Here's how the part is built. I have some questions about the finished solid (model axes, mm). Face numbers are marked on the shaded views. A direction names the side the tool comes from. Round coordinates to 2 decimals unless told otherwise and drop trailing zeros. Loops run counter-clockwise (first coordinate to the right, second up) from the corner with the lowest first, then second, coordinate; pieces in that order, holes last. Notation, with made-up numbers: M 40,22 L 92,22 A29 cw 92,51 Z; hole C -8.75,-9.75 d4. An arc over 180 degrees is marked long. Use a Markdown table: item, result.
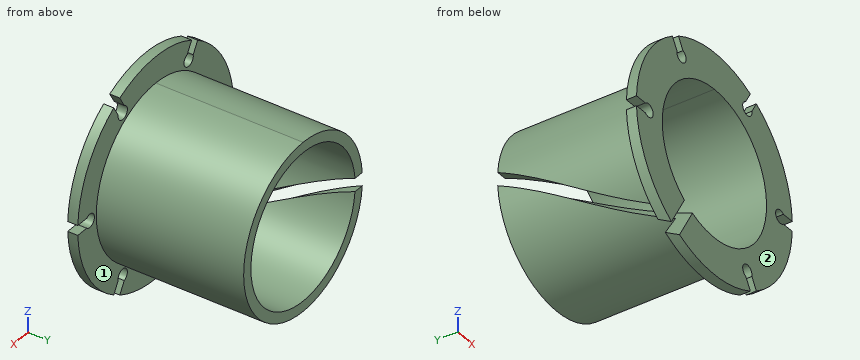
from build123d import *

# Parameters (mm, degrees)
SKETCH2_R           = 6.35
SKETCH2_R_2         = 5.5753
BOSS_EXTRUDE1_DEPTH = 11.8872
SKETCH3_R           = 8.334375
SKETCH3_R_2         = 6.35
BOSS_EXTRUDE2_DEPTH = 0.762
CUT_EXTRUDE1_DEPTH  = 17.207827995
CIRPATTERN1_COUNT   = 6


with BuildPart() as part:
    # Sketch2 → Boss-Extrude1 (new body)
    with BuildSketch(Plane(origin=(0, 0, 0), x_dir=(1, 0, 0), z_dir=(0, 1, 0))):
        with Locations(Location((0, 0, 0), (0, 0, 270))):
            Circle(SKETCH2_R)
        with Locations(Location((0, 0, 0), (0, 0, 270))):
            Circle(SKETCH2_R_2, mode=Mode.SUBTRACT)
    extrude(amount=BOSS_EXTRUDE1_DEPTH)

    # Sketch3 → Boss-Extrude2 (add)
    with BuildSketch(Plane(origin=(0, 0, 0), x_dir=(1, 0, 0), z_dir=(0, 1, 0))):
        with Locations(Location((0, 0, 0), (0, 0, 90))):
            Circle(SKETCH3_R)
        with Locations(Location((0, 0, 0), (0, 0, 270))):
            Circle(SKETCH3_R_2, mode=Mode.SUBTRACT)
    extrude(amount=BOSS_EXTRUDE2_DEPTH)

    # Sketch7 → Cut-Extrude1 (cut, through all)
    with BuildSketch(Plane(origin=(0, 0.762, 0), x_dir=(1, 0, 0), z_dir=(0, 1, 0))):
        with BuildLine():
            Line((-7.372666422, 0.372070313), (-8.334375, 0.372070312))
            Line((-8.334375, 0.372070312), (-8.334375, -0.372070312))
            Line((-8.334375, -0.372070312), (-7.372666422, -0.372070313))
            ThreePointArc((-7.372666422, -0.372070313), (-6.5484375, 0), (-7.372666422, 0.372070313))
        make_face()
    cut_extrude1 = extrude(amount=-CUT_EXTRUDE1_DEPTH, mode=Mode.SUBTRACT)

    # CirPattern1: Cut-Extrude1 ×6 about axis, 1 skipped
    cirpattern1_axis = Axis((0, 11.8872, 0), (0, -1, 0))
    add([cut_extrude1.rotate(cirpattern1_axis, i * 360 / CIRPATTERN1_COUNT) for i in range(1, CIRPATTERN1_COUNT) if i not in (1,)], mode=Mode.SUBTRACT)

    # Sketch13 → Cut-Loft1 section 0
    with BuildSketch(Plane.XZ):
        with BuildLine():
            Line((-3.206222175, -4.561152207), (-5.86681729, -9.169438125))
            Line((-5.86681729, -9.169438125), (-5.00755771, -9.665531875))
            Line((-5.00755771, -9.665531875), (-2.346962594, -5.057245957))
            Line((-2.346962594, -5.057245957), (-3.206222175, -4.561152207))
        make_face()
    # Sketch12 → Cut-Loft1 section 1
    with BuildSketch(Plane(origin=(0, 11.8872, 0), x_dir=(1, 0, 0), z_dir=(0, 1, 0))):
        with BuildLine():
            Line((-10.874375, 0.49609375), (-5.553184769, 0.49609375))
            Line((-5.553184769, 0.49609375), (-5.553184769, -0.49609375))
            Line((-5.553184769, -0.49609375), (-10.874375, -0.49609375))
            Line((-10.874375, -0.49609375), (-10.874375, 0.49609375))
        make_face()
    loft(mode=Mode.SUBTRACT)


solid = part.part
1. I need wall thicknesses on probe 1 along Z at (x, y) = (-0.25, 11.25); probe 2 along X at (y, z) = (0.25, 0); probe 3 along Y at (x, z) = (-1.5, -7.5). Which ranges of each line are inside material? Lowest first, please. Write a range as from..to.
Answer sheet:
| item | result |
|---|---|
| probe 1 | -6.35..-5.57, 5.57..6.35 |
| probe 2 | -6.55..-5.58, 5.58..6.55 |
| probe 3 | 0..0.76 |
2. Which directions (+Z, -Z, +X, -X, +Y, -Y) give clear straight access to the entire face, cutting with the end or side of a thin tool? Please do the marked faces 1 and 2.
Answer sheet:
| item | result |
|---|---|
| face 1 | +Y |
| face 2 | +Z, -Z, +X, -X, -Y |
3. Imagine slicing it at A-A, the plane x = 0.75. Write out the boundary of the cut face in (y, z).
Answer sheet:
| item | result |
|---|---|
| outline | M 0,-8.3 L 0.76,-8.3 L 0.76,-6.31 L 11.89,-6.31 L 11.89,-5.52 L 0,-5.52 Z; M 0,5.52 L 11.89,5.52 L 11.89,6.31 L 0.76,6.31 L 0.76,8.3 L 0,8.3 Z |
4. For pin 1 Ø6 at (x, z) = (-5, 2) entering from -Y; pin 2 Ø6 at (y, z) = (2, -6.5) entering from +X; pin 3 Ø5 at (x, y) = (-1.5, 4.5) entering from -Z; pin 4 Ø0.8 at (x, y) = (8, 0.5) entering from -Z, each with a flat end and sliding along its axis, tell me the tip position at first contact or that it passes through.
Answer sheet:
| item | result |
|---|---|
| pin 1 | y = 0 |
| pin 2 | x = 7.43 |
| pin 3 | z = -6.35 |
| pin 4 | z = -3.42 |
5. Imagine slicing it at B-B, the plane z = -0.75. State how many separate pieces and enclosed holes the cut face has, then the cut area to 3 significant figures.
Answer sheet:
| item | result |
|---|---|
| separate pieces | 3 |
| enclosed holes | 0 |
| area | 20.1 mm2 |
